Check sheet for the modelled part. Datum: model origin and axes. Units: mm. A direction names the side the tool comes from. Give positions to 0.01 mm unless a question says otherwise; leave off trailing zeros. Order: outer loops, then holes, each group sorted by start corner. A loop starts at its lowest first (then second) coordinate and runs counter-clockwise, first axis right, second up.
Item 1: Sectioned sample at B-B on z = 300. Record the boundary of the cut face in (x, y), and give its area (3 significant figures).
Item 2: Sectioned sample at A-A on y = -9. Record the boundary of the cut face in (x, z).
Item 3: Material ranges on line 1 along X through (y, z) = (-15.25, 277.5), recorded low to high.
Item 4: Access from +Z, -Z, +X, -X, +Y, -Y to the whole of each face (thin tool, end or side, straight path). Record for faces 1 (the flat face through (-65.788, -9, 22)), 2 (the flat face through (-47.5, -9, 222)), 3 (the flat face through (611, -9, 59.734)), 4 (the flat face through (-57, -9, -16.466)), 5 (the flat face through (611, -9, -16.466)).
Item 5: Gauge pin test, flat ends, axial feed: P1, Ø5.5, axis at y = -8.5, z = 275.5, coming from the +X side; P2, Ø5.5, axis at x = 610, y = -7, coming from the -Z side; P3, Ø1.5, axis at x = 212.5, z = 157, coming from the +Y side; P4, Ø8.5, axis at y = -7, z = -21.5, coming from the -X side. Record the tip position at first contact, or that the pin passes through.
from build123d import *

# Parameters (mm, degrees)
F0_W     = 18.288
F0_H     = 76.2
F1_DEPTH = 18.288


with BuildPart() as f1:
    # F0 (on Front) → F1 (new body)
    with BuildSketch(Plane.XZ):
        Polygon((601.724416, 379.273323), (-47.499584, 379.273323), (-47.499584, 59.734055), (-47.499584, -16.465945), (-47.499584, -27.126677), (601.724416, -27.126677), (601.724416, -16.465945), (601.724416, 59.734055), align=None)
        Polygon((-47.499584, -16.465945), (-47.499584, 59.734055), (-65.787584, 59.734055), (-65.787584, 21.634055), (-65.787584, -5.497572), (-65.787584, -16.465945), align=None)
        with Locations((610.868416, 21.634055)):
            Rectangle(F0_W, F0_H)
    extrude(amount=F1_DEPTH)


solid = f1.part
Report:
1. outline: (-47.5, -18.29) - (601.72, -18.29) - (601.72, 0) - (-47.5, 0) - close
1. area: 11,900 mm2
2. outline: (-65.79, -16.47) - (-47.5, -16.47) - (-47.5, -27.13) - (601.72, -27.13) - (601.72, -16.47) - (620.01, -16.47) - (620.01, 59.73) - (601.72, 59.73) - (601.72, 379.27) - (-47.5, 379.27) - (-47.5, 59.73) - (-65.79, 59.73) - close
3. line 1: x = -47.5 to 601.72
4. face 1: +Z, -Z, -X, +Y, -Y
4. face 2: +Z, -X, +Y, -Y
4. face 3: +Z, +X, +Y, -Y
4. face 4: -Z, -X, +Y, -Y
4. face 5: -Z, +X, +Y, -Y
5. P1: stops at x = 601.72
5. P2: stops at z = -16.47
5. P3: stops at y = 0
5. P4: stops at x = -47.5
